Here's how the part is built. I have some questions about the finished solid (model axes, mm). A direction names the side the tool comes from. Give positions to 0.01 mm unless a question says otherwise; leave off trailing zeros. Loops run counter-clockwise (first coordinate to the right, second up) from the corner with the lowest first, then second, coordinate; pieces in that order, holes last. Notation, with made-up numbers: (-9, 59.5) - (7, 59.5) arc R7 cw to (7, 67.5) - close; hole circle Ø6 at (-40, 39.25). An arc over 180 degrees is marked (long way). One line per item, written item: value. Start each with the question number.
```python
from build123d import *

# Parameters (mm, degrees)
BOSS_EXTRUDE1_DEPTH = 10
SKETCH3_R           = 2.5
CUT_EXTRUDE1_DEPTH  = 10
BOSS_EXTRUDE2_DEPTH = 5


with BuildPart() as part:
    # Sketch1 → Boss-Extrude1 (new body)
    with BuildSketch(Plane(origin=(0, 0, 0), x_dir=(1, 0, 0), z_dir=(0, 1, 0))):
        with BuildLine():
            Line((62.5, 6), (31.941352507, 6))
            ThreePointArc((31.941352507, 6), (0, 32.5), (-31.941352507, 6))
            Line((-31.941352507, 6), (-47.5, 6))
            Line((-47.5, 6), (-47.5, 0))
            Line((-47.5, 0), (-30, 0))
            ThreePointArc((-30, 0), (0, 30), (30, 0))
            Line((30, 0), (62.5, 0))
            Line((62.5, 0), (62.5, 6))
        make_face()
    extrude(amount=BOSS_EXTRUDE1_DEPTH)

    # Sketch3 → Cut-Extrude1 (cut)
    with BuildSketch(Plane.XY):
        with Locations((57.5, 5)):
            Circle(SKETCH3_R)
        with Locations((-42.5, 5)):
            Circle(SKETCH3_R)
    extrude(amount=-CUT_EXTRUDE1_DEPTH, mode=Mode.SUBTRACT)

    # Sketch5 → Boss-Extrude2 (add)
    with BuildSketch(Plane(origin=(0, 0, 0), x_dir=(1, 0, 0), z_dir=(0, 1, 0))):
        with BuildLine():
            ThreePointArc((37.5, 0), (0, 37.5), (-37.5, 0))
            Line((-37.5, 0), (-32.5, 0))
            ThreePointArc((-32.5, 0), (0, 32.5), (32.5, 0))
            Line((32.5, 0), (37.5, 0))
        make_face()
    extrude(amount=BOSS_EXTRUDE2_DEPTH)


solid = part.part
```
(1) If we section it at A-A on y = 3.5: List the corners of the cut face in (x, z) for me, plus the area to 3 significant figures.
(2) If we section it at B-B on x = 57.5: List the corners of the cut face in (y, z) for me.
(3) If we section it at C-C on z = -9: List the corners of the cut face in (x, y) for me, plus the area to 3 significant figures.
(4) For faces 4 (the face through (15.4, 10, -26)), 5 (the face through (-39.6, 4.9, -6)), 6 (the face through (0.63, 7.465, -32.494)), which set-ups out of +Z, -Z, +X, -X, +Y, -Y let a thin tool reach every point of the face, with its end or its side?
(5) Please list where these lines run through material, in increasing order: probe 1 along Y at (x, z) = (57.5, -1.45); probe 2 along X at (y, z) = (3.75, -12.5); probe 3 along X at (y, z) = (2.5, -22.5). Write a range as from..to.
(6) Will these pins go through, and if not, where does the flat tip stop? pin 1 (1 mm diameter, centred on y = 4.5, z = -18, fed in from +X); pin 2 (3 mm diameter, centred on x = 52, y = 7, fed in from -Z); pin 3 (2 mm diameter, centred on x = 21.5, y = 3.5, fed in from -Z); pin 4 (4.5 mm diameter, centred on x = -42.5, y = 5, fed in from +Z).
(7) If we mould it in two halves opening along Y, with no side actions, what happens to faces 1 (the face through (11, 0, -29)), 2 (the face through (-40.19, 4.04, -2.96)), 3 (the face through (0.74, 2.465, -37.493))? For each: pulls with the +Y half, pulls with the -Y half, needs draft (parallel to the pull), parting line crosses it, or undercut.
(8) If we section it at D-D on y = 9: List the corners of the cut face in (x, z) for me.
Found:
1. outline: (-47.5, -6) - (-44.5, -6) - (-44.5, 0) - (-47.5, 0) - close; (-40.5, -6) - (-37.02, -6) arc R37.5 ccw to (37.02, -6) - (55.5, -6) - (55.5, 0) - (30, 0) arc R30 cw to (-30, 0) - (-40.5, 0) - close; (59.5, -6) - (62.5, -6) - (62.5, 0) - (59.5, 0) - close
1. area: 959 mm^2
2. outline: (0, -6) - (2.5, -6) - (2.5, 0) - (0, 0) - close; (7.5, -6) - (10, -6) - (10, 0) - (7.5, 0) - close
3. outline: (-36.4, 0) - (-28.62, 0) - (-28.62, 10) - (-31.23, 10) - (-31.23, 5) - (-36.4, 5) - close; (28.62, 0) - (36.4, 0) - (36.4, 5) - (31.23, 5) - (31.23, 10) - (28.62, 10) - close
3. area: 104 mm^2
4. face 4: +Z, -Z, +X, -X, +Y
4. face 5: -Z, -X, +Y
4. face 6: -Z, +Y
5. probe 1: 0..2.5, 7.5..10
5. probe 2: -35.36..-27.27, 27.27..35.36
5. probe 3: -30..-19.84, 19.84..30
6. pin 1: x = 33.17
6. pin 2: z = -6
6. pin 3: z = -31.4
6. pin 4: through
7. face 1: pulls with the -Y half
7. face 2: undercut
7. face 3: needs draft
8. outline: (-47.5, -6) - (-31.94, -6) arc R32.5 ccw to (31.94, -6) - (62.5, -6) - (62.5, 0) - (30, 0) arc R30 cw to (-30, 0) - (-47.5, 0) - close
